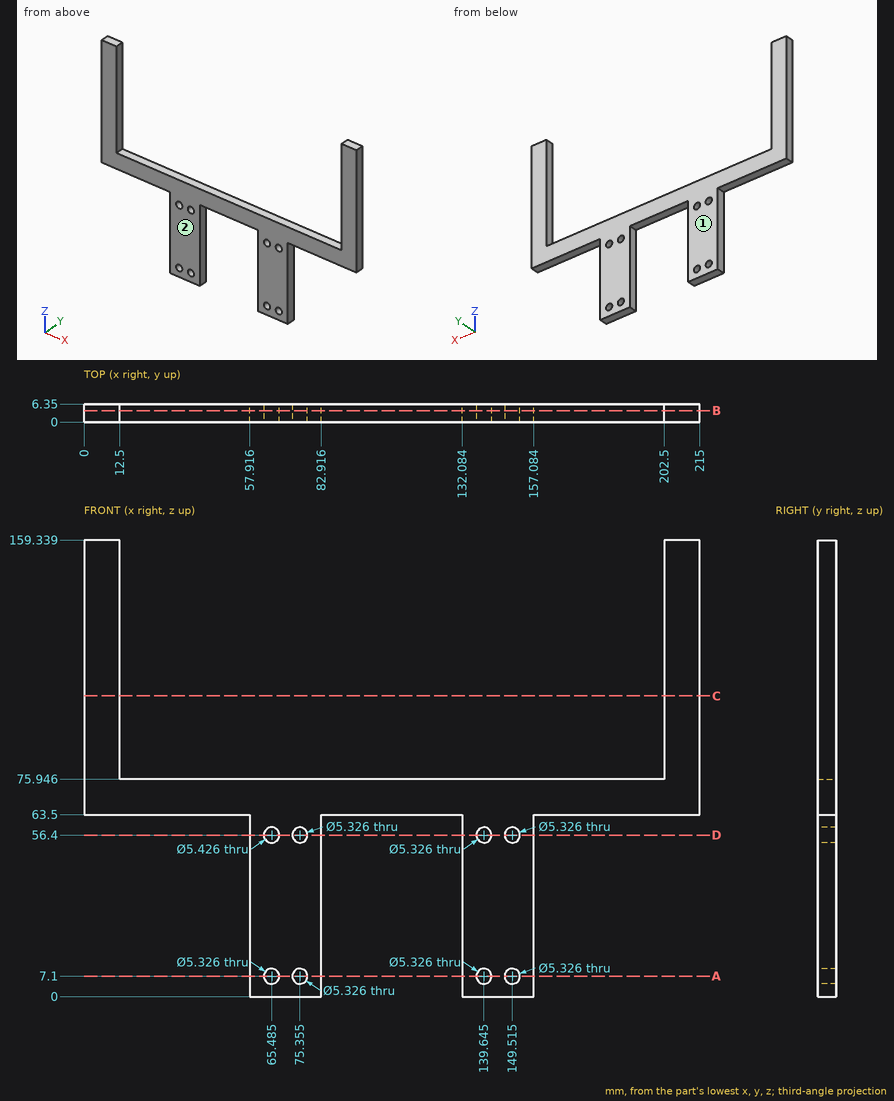
Print and shaded views of the part. All mm, measured from the part's lowest x, y and z. Round coordinates to 2 decimals unless told otherwise and drop trailing zeros. Order: outer loops, then holes, each group sorted by start corner. A loop starts at its lowest first (then second) coordinate and runs counter-clockwise, first axis right, second up.
Q1. Slice it at C-C (z = 105). Write the cut outline in (x, y), and give its area (3 significant figures).
Q2. Two-plate mould, pull along Y, no slides. Class the marked faces 1 and 2: pulls with the +Y half, pulls with the -Y half, needs draft (parallel to the pull), parting line crosses it, or undercut.
Q3. Wall check: L1, parallel to Z at x = 149, y = 5.75 (1 decimal); L2, parallel to X at y = 5, z = 38.5; L3, parallel to X at y = 1.5, z = 117.5. Give the ranges that are in metal, low to high.
Q4. Drop flat-ended pins along their axis: pin 1 (2 mm diameter, centred on y = 1.5, z = 61.5, fed in from -X); pin 2 (1.9 mm diameter, centred on x = 101, y = 3.5, fed in from +Z); pin 3 (3 mm diameter, centred on x = 106.5, y = 4.5, fed in from -Z). Give the stop position or say it passes through.
Q5. Slice it at B-B (y = 4). State how many separate pieces and enclosed holes the cut face has, and give its area (3 significant figures).
Q6. Slice it at A-A (z = 7.1). Write the cut outline in (x, y), and give its area (3 significant figures).
Q7. Slice it at D-D (z = 56.4). Write the cut outline in (x, y).
Results below:
1. outline: (0, 0) - (12.5, 0) - (12.5, 6.35) - (0, 6.35) - close; (202.5, 0) - (215, 0) - (215, 6.35) - (202.5, 6.35) - close
1. area: 159 mm2
2. face 1: pulls with the +Y half
2. face 2: pulls with the -Y half
3. L1: z = 0 to 4.5, 9.7 to 53.8, 59 to 75.9
3. L2: x = 57.92 to 82.92, 132.08 to 157.08
3. L3: x = 0 to 12.5, 202.5 to 215
4. pin 1: stops at x = 57.92
4. pin 2: stops at z = 75.95
4. pin 3: stops at z = 63.5
5. separate pieces: 1
5. enclosed holes: 8
5. area: 7,760 mm2
6. outline: (57.92, 0) - (62.82, 0) - (62.82, 6.35) - (57.92, 6.35) - close; (68.15, 0) - (72.69, 0) - (72.69, 6.35) - (68.15, 6.35) - close; (78.02, 0) - (82.92, 0) - (82.92, 6.35) - (78.02, 6.35) - close; (132.08, 0) - (136.98, 0) - (136.98, 6.35) - (132.08, 6.35) - close; (142.31, 0) - (146.85, 0) - (146.85, 6.35) - (142.31, 6.35) - close; (152.18, 0) - (157.08, 0) - (157.08, 6.35) - (152.18, 6.35) - close
6. area: 182 mm2
7. outline: (57.92, 0) - (62.77, 0) - (62.77, 6.35) - (57.92, 6.35) - close; (68.2, 0) - (72.69, 0) - (72.69, 6.35) - (68.2, 6.35) - close; (78.02, 0) - (82.92, 0) - (82.92, 6.35) - (78.02, 6.35) - close; (132.08, 0) - (136.98, 0) - (136.98, 6.35) - (132.08, 6.35) - close; (142.31, 0) - (146.85, 0) - (146.85, 6.35) - (142.31, 6.35) - close; (152.18, 0) - (157.08, 0) - (157.08, 6.35) - (152.18, 6.35) - close
